```python
from build123d import *

# Parameters (mm, degrees)
F1_DEPTH = 30
F2_DEPTH = 15


with BuildPart() as f1:
    # F0 (on Top) → F1 (new body)
    with BuildSketch(Plane.XY):
        with BuildLine():
            Line((80, 0), (0, 0))
            Line((0, 0), (0, -80))
            Line((0, -80), (20, -80))
            Line((20, -80), (20, -54.806759))
            ThreePointArc((20, -54.806759), (28.786797, -33.593555), (50, -24.806759))
            Line((50, -24.806759), (80, -24.806759))
            Line((80, -24.806759), (80, 0))
        make_face()
        with BuildLine():
            Line((80, -50), (80, -24.806759))
            Line((80, -24.806759), (50, -24.806759))
            ThreePointArc((50, -24.806759), (28.786797, -33.593555), (20, -54.806759))
            Line((20, -54.806759), (20, -80))
            Line((20, -80), (60, -80))
            ThreePointArc((60, -80), (66.428126, -62.618751), (80, -50))
        make_face()
        with BuildLine():
            Line((80, -80), (80, -50))
            ThreePointArc((80, -50), (66.428126, -62.618751), (60, -80))
            Line((60, -80), (80, -80))
        make_face()
    extrude(amount=-F1_DEPTH)

    # F0 (on Top) → F2 (cut)
    with BuildSketch(Plane.XY):
        with BuildLine():
            Line((80, -50), (80, -24.806759))
            Line((80, -24.806759), (50, -24.806759))
            ThreePointArc((50, -24.806759), (28.786797, -33.593555), (20, -54.806759))
            Line((20, -54.806759), (20, -80))
            Line((20, -80), (60, -80))
            ThreePointArc((60, -80), (66.428126, -62.618751), (80, -50))
        make_face()
    extrude(amount=-F2_DEPTH, mode=Mode.SUBTRACT)


solid = f1.part
```
Part model, mm, in its own coordinate system. A direction names the side the tool comes from. Coordinates: 2 decimals unless noted, no trailing zeros. Loops run counter-clockwise (first coordinate to the right, second up) from the corner with the lowest first, then second, coordinate; pieces in that order, holes last. Notation, with made-up numbers: (67.25, -35) - (76.25, -35) arc R21 cw to (76.25, -29) - close; hole circle Ø6 at (-32.5, 26). An arc over 180 degrees is marked (long way). Write item = value, one per line. Start each with the question number.
Item 1: Cut at B-B, the plane y = -64. Give the cut face in (x, z).
Item 2: Cut at D-D, the plane x = 53. Give the cut face in (y, z).
Item 3: Cut at C-C, the plane x = 61. Give the cut face in (y, z).
Item 4: Flat gauge pins, fed straight in: pin 1 Ø8 at (x, y) = (62, -47.5) entering from +Z; pin 2 Ø3 at (x, z) = (55.5, -12) entering from -Y. Where does each tip first touch, or does it go through?
Item 5: Cut at A-A, the plane z = -3. Give the cut face in (x, y), and give its area (3 significant figures).
Item 6: 3-axis set-ups, long thin cutter, end or side, ignore diameter. For faces 1 (the flat face through (20, -67, -7)), 2 (the flat face through (65, -24.807, -7)), 3 (the cylindrical face through (66.28, -62.84, -7.4)): which of +Z, -Z, +X, -X, +Y, -Y reach the whole face in a straight line?
Item 7: Wall check: L1, parallel to Z at x = 21, y = -73; L2, parallel to X at y = -64.5, z = -2.5; L3, parallel to Y at x = 63, z = -12. Give the ranges that are in metal, low to high. Write a range as from..to.
The answers:
q1.outline = (0, -30) - (80, -30) - (80, 0) - (65.55, 0) - (65.55, -15) - (20, -15) - (20, 0) - (0, 0) - close
q2.outline = (-80, -30) - (0, -30) - (0, 0) - (-24.81, 0) - (-24.81, -15) - (-80, -15) - close
q3.outline = (-80, -30) - (0, -30) - (0, 0) - (-24.81, 0) - (-24.81, -15) - (-74.73, -15) - (-74.73, 0) - (-80, 0) - close
q4.pin_1 = -15
q4.pin_2 = -24.81
q5.outline = (0, -80) - (20, -80) - (20, -54.81) arc R30 cw to (50, -24.81) - (80, -24.81) - (80, 0) - (0, 0) - close; (60, -80) - (80, -80) - (80, -50) arc R40 ccw to start
q5.area = 3,690 mm2
q6.face_1 = +Z, -Y
q6.face_2 = +Z, +X
q6.face_3 = +Z
q7.L1 = -30..-15
q7.L2 = 0..20, 65.25..80
q7.L3 = -80..-68.92, -24.81..0
